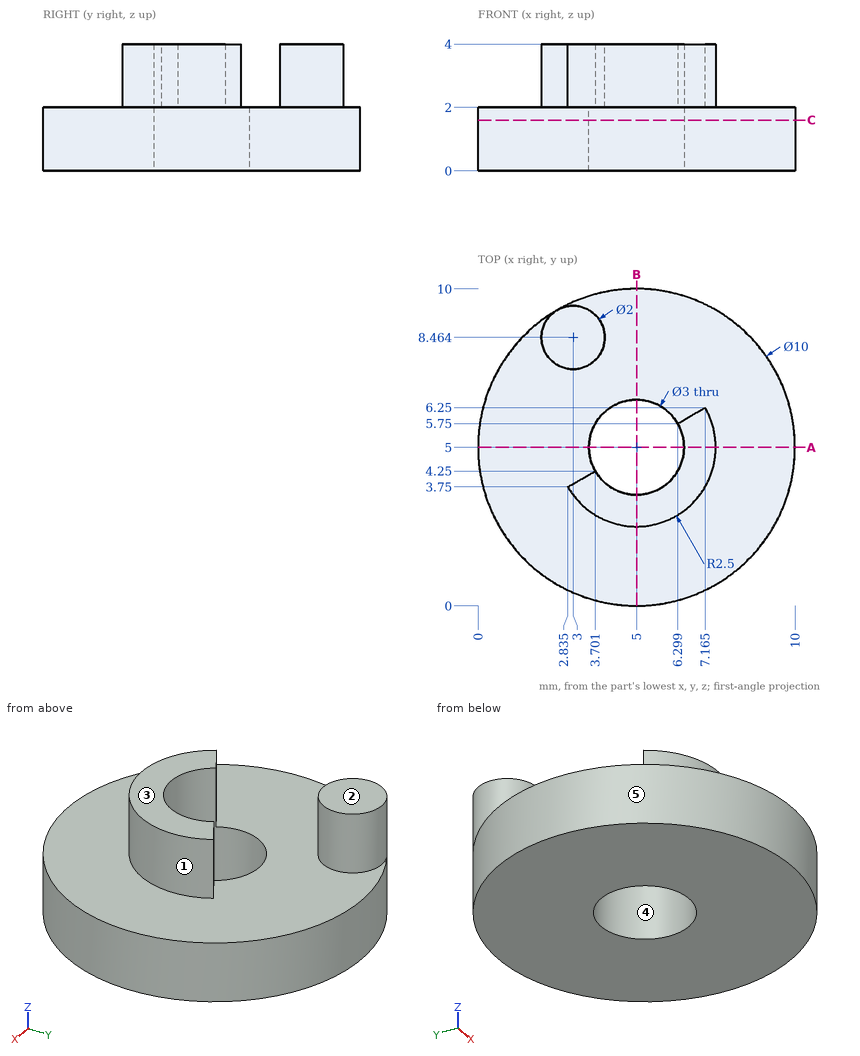
Here's the drawing with two shaded views (mm, measured from the low corner). I have some questions. A direction names the side the tool comes from. Give positions to 0.01 mm unless a question says otherwise; leave off trailing zeros. Order: outer loops, then holes, each group sorted by start corner. A loop starts at its lowest first (then second) coordinate and runs counter-clockwise, first axis right, second up. Notation, with made-up numbers: (-23.75, 41) -> (6.25, 41) arc R36 cw to (6.25, 79) -> close; hole circle Ø6 at (60, 71.5). An arc over 180 degrees is marked (long way). Use a Markdown table: item, result. Add a question column.
Item 1: Imagine slicing it at B-B on x = 5. Please give me the cut outline in (y, z).
Item 2: Imagine slicing it at C-C on z = 1.6. Please give me the cut outline in (x, y).
Item 3: For the marked faces 1 and 2, which set-ups out of +Z, -Z, +X, -X, +Y, -Y let a thin tool reach every point of the face, with its end or its side?
Item 4: If we mould it in two halves opening along Y, with no side actions, what happens to the marked faces 3, 4 and 5? For each: pulls with the +Y half, pulls with the -Y half, needs draft (parallel to the pull), parting line crosses it, or undercut.
Item 5: Will these pins go through, and if not, where does the flat tip stop? pin 1 (1.5 mm diameter, centred on x = 4, y = 6, fed in from +Z); pin 2 (2 mm diameter, centred on y = 4, z = 2.5, fed in from +X); pin 3 (1 mm diameter, centred on x = 6, z = 0.5, fed in from -Y) (3 decimals).
Item 6: I need wall thicknesses on line 1 (Y direction, x = 5, z = 1.15); line 2 (Z direction, x = 8.5, y = 3). Which ranges of each line are inside material? Lowest first, please.
Item 7: Imagine slicing it at A-A on y = 5. Please give me the cut outline in (x, z).
Data:
| question | item | result |
|---|---|---|
| 1 | outline | (0, 0) -> (3.5, 0) -> (3.5, 4) -> (2.5, 4) -> (2.5, 2) -> (0, 2) -> close; (6.5, 0) -> (10, 0) -> (10, 2) -> (6.5, 2) -> close |
| 2 | outline | circle Ø10 at (5, 5); hole circle Ø3 at (5, 5) |
| 3 | face 1 | +Z |
| 3 | face 2 | +Z, +X, -X, +Y, -Y |
| 4 | face 3 | needs draft |
| 4 | face 4 | undercut |
| 4 | face 5 | parting line crosses it |
| 5 | pin 1 | stops at z = 2 |
| 5 | pin 2 | stops at x = 10 |
| 5 | pin 3 | stops at y = 0.025 |
| 6 | line 1 | y = 0 to 3.5, 6.5 to 10 |
| 6 | line 2 | z = 0 to 2 |
| 7 | outline | (0, 0) -> (3.5, 0) -> (3.5, 2) -> (0, 2) -> close; (6.5, 0) -> (10, 0) -> (10, 2) -> (7.5, 2) -> (7.5, 4) -> (6.5, 4) -> close |
